from build123d import *

# Parameters (mm, degrees)
SKETCH1_W           = 60
SKETCH1_H           = 25
BOSS_EXTRUDE1_DEPTH = 4
SKETCH3_R           = 1.6
CUT_EXTRUDE1_DEPTH  = 66.122960621
SKETCH4_W           = 60
SKETCH4_H           = 25
SKETCH4_W_2         = 24
SKETCH4_H_2         = 19
SKETCH4_W_3         = 27
BOSS_EXTRUDE2_DEPTH = 30
SKETCH5_R           = 5.25
CUT_EXTRUDE2_DEPTH  = 74.35529974
CUT_EXTRUDE3_REACH  = 75.355
SKETCH6_R           = 1.6
FILLET3_R           = 3
FILLET4_R           = 1
FILLET5_R           = 6
CUT_EXTRUDE4_DEPTH  = 74.35529974
CUT_EXTRUDE5_REACH  = 75.355
CUT_EXTRUDE6_REACH  = 75.355


with BuildPart() as part:
    # Sketch1 → Boss-Extrude1 (new body)
    with BuildSketch(Plane(origin=(0, 0, 0), x_dir=(1, 0, 0), z_dir=(0, 1, 0))):
        with Locations((30, 12.5)):
            Rectangle(SKETCH1_W, SKETCH1_H)
    extrude(amount=BOSS_EXTRUDE1_DEPTH)

    # Sketch3 → Cut-Extrude1 (cut, through all)
    with BuildSketch(Plane(origin=(0, 4, 0), x_dir=(1, 0, 0), z_dir=(0, 1, 0))):
        with Locations(Location((7.5, 17.5, 0), (0, 0, 270))):
            Circle(SKETCH3_R)
        with Locations(Location((22.5, 17.5, 0), (0, 0, 270))):
            Circle(SKETCH3_R)
        with Locations(Location((22.5, 7.5, 0), (0, 0, 270))):
            Circle(SKETCH3_R)
        with Locations(Location((7.5, 7.5, 0), (0, 0, 270))):
            Circle(SKETCH3_R)
    extrude(amount=-CUT_EXTRUDE1_DEPTH, mode=Mode.SUBTRACT)

    # Sketch4 → Boss-Extrude2 (add)
    with BuildSketch(Plane(origin=(0, 4, 0), x_dir=(1, 0, 0), z_dir=(0, 1, 0))):
        with Locations((30, 12.5)):
            Rectangle(SKETCH4_W, SKETCH4_H)
        with Locations((15, 12.5)):
            Rectangle(SKETCH4_W_2, SKETCH4_H_2, mode=Mode.SUBTRACT)
        with Locations((43.5, 12.5)):
            Rectangle(SKETCH4_W_3, SKETCH4_H_2, mode=Mode.SUBTRACT)
    extrude(amount=BOSS_EXTRUDE2_DEPTH)

    # Sketch5 → Cut-Extrude2 (cut, through all)
    with BuildSketch(Plane(origin=(0, 0, -25), x_dir=(-1, 0, 0), z_dir=(0, 0, -1))):
        with Locations((-43.5, 20)):
            Circle(SKETCH5_R)
    extrude(amount=-CUT_EXTRUDE2_DEPTH, mode=Mode.SUBTRACT)

    # Sketch6 → Cut-Extrude3 (cut, up to next)
    with BuildSketch(Plane(origin=(0, 0, -25), x_dir=(-1, 0, 0), z_dir=(0, 0, -1)), mode=Mode.PRIVATE) as cut_extrude3_sk1:
        with Locations((-37.843145751, 14.343145751)):
            Circle(SKETCH6_R)
    cut_extrude3_tool1 = extrude(cut_extrude3_sk1.sketch, amount=-CUT_EXTRUDE3_REACH, mode=Mode.PRIVATE) & part.part
    # Sketch6 → Cut-Extrude3 (cut, up to next)
    with BuildSketch(Plane(origin=(0, 0, -25), x_dir=(-1, 0, 0), z_dir=(0, 0, -1)), mode=Mode.PRIVATE) as cut_extrude3_sk2:
        with Locations((-49.156854249, 14.343145751)):
            Circle(SKETCH6_R)
    cut_extrude3_tool2 = extrude(cut_extrude3_sk2.sketch, amount=-CUT_EXTRUDE3_REACH, mode=Mode.PRIVATE) & part.part
    # Sketch6 → Cut-Extrude3 (cut, up to next)
    with BuildSketch(Plane(origin=(0, 0, -25), x_dir=(-1, 0, 0), z_dir=(0, 0, -1)), mode=Mode.PRIVATE) as cut_extrude3_sk3:
        with Locations((-49.156854249, 25.656854249)):
            Circle(SKETCH6_R)
    cut_extrude3_tool3 = extrude(cut_extrude3_sk3.sketch, amount=-CUT_EXTRUDE3_REACH, mode=Mode.PRIVATE) & part.part
    # Sketch6 → Cut-Extrude3 (cut, up to next)
    with BuildSketch(Plane(origin=(0, 0, -25), x_dir=(-1, 0, 0), z_dir=(0, 0, -1)), mode=Mode.PRIVATE) as cut_extrude3_sk4:
        with Locations((-37.843145751, 25.656854249)):
            Circle(SKETCH6_R)
    cut_extrude3_tool4 = extrude(cut_extrude3_sk4.sketch, amount=-CUT_EXTRUDE3_REACH, mode=Mode.PRIVATE) & part.part
    add(cut_extrude3_tool1.solids().sort_by_distance((37.843146, 14.343146, -25))[0], mode=Mode.SUBTRACT)
    add(cut_extrude3_tool2.solids().sort_by_distance((49.156854, 14.343146, -25))[0], mode=Mode.SUBTRACT)
    add(cut_extrude3_tool3.solids().sort_by_distance((49.156854, 25.656854, -25))[0], mode=Mode.SUBTRACT)
    add(cut_extrude3_tool4.solids().sort_by_distance((37.843146, 25.656854, -25))[0], mode=Mode.SUBTRACT)

    # Fillet3
    fillet3_edges = [part.edges().sort_by_distance(p)[0] for p in [
        (3, 19, -3),
        (27, 19, -3),
        (27, 19, -22),
        (3, 19, -22),
        (57, 19, -3),
        (57, 19, -22),
        (30, 19, -22),
        (30, 19, -3),
    ]]
    fillet(fillet3_edges, radius=FILLET3_R)

    # Fillet4
    fillet4_edges = [part.edges().sort_by_distance(p)[0] for p in [
        (15, 4, -3),
        (15, 4, -22),
        (3, 4, -12.5),
        (27, 4, -12.5),
        (26.121320344, 4, -21.121320344),
        (3.878679656, 4, -21.121320344),
        (3.878679656, 4, -3.878679656),
        (26.121320344, 4, -3.878679656),
        (30, 4, -12.5),
        (43.5, 4, -3),
        (57, 4, -12.5),
        (43.5, 4, -22),
        (30.878679656, 4, -21.121320344),
        (56.121320344, 4, -21.121320344),
        (56.121320344, 4, -3.878679656),
        (30.878679656, 4, -3.878679656),
    ]]
    fillet(fillet4_edges, radius=FILLET4_R)

    # Fillet5
    fillet5_edges = [part.edges().sort_by_distance(p)[0] for p in [
        (0, 17, -25),
        (60, 17, -25),
        (60, 17, 0),
        (0, 17, 0),
    ]]
    fillet(fillet5_edges, radius=FILLET5_R)

    # Sketch7 → Cut-Extrude4 (cut, through all)
    with BuildSketch(Plane(origin=(0, 0, -25), x_dir=(-1, 0, 0), z_dir=(0, 0, -1))):
        with BuildLine():
            Line((-13.4, 26), (-13.4, 34))
            Line((-13.4, 34), (-16.6, 34))
            Line((-16.6, 34), (-16.6, 26))
            ThreePointArc((-16.6, 26), (-15, 24.4), (-13.4, 26))
        make_face()
    extrude(amount=-CUT_EXTRUDE4_DEPTH, mode=Mode.SUBTRACT)

    # Cut-Extrude5: up to this face of the body (flat: up to its plane)
    cut_extrude5_end = Plane(part.part.faces().sort_by_distance((30, 19.5, -12.5))[0])
    # Sketch8 → Cut-Extrude5 (cut, up to the picked face)
    with BuildSketch(Plane.ZY, mode=Mode.PRIVATE) as cut_extrude5_sk1:
        with BuildLine():
            Line((-14.1, 26), (-14.1, 34))
            Line((-14.1, 34), (-10.9, 34))
            Line((-10.9, 34), (-10.9, 26))
            ThreePointArc((-10.9, 26), (-12.5, 24.4), (-14.1, 26))
        make_face()
    cut_extrude5_tool1 = split(extrude(cut_extrude5_sk1.sketch, amount=-CUT_EXTRUDE5_REACH, mode=Mode.PRIVATE), bisect_by=cut_extrude5_end, keep=Keep.BOTH, mode=Mode.PRIVATE)
    add(cut_extrude5_tool1.solids().sort_by(Axis((0, 29.364793, -12.5), (1, 0, 0)))[0], mode=Mode.SUBTRACT)

    # Sketch9 → Cut-Extrude6 (cut, up to next)
    with BuildSketch(Plane(origin=(60, 0, 0), x_dir=(0, 0, -1), z_dir=(1, 0, 0)), mode=Mode.PRIVATE) as cut_extrude6_sk1:
        with BuildLine():
            Line((15, 29), (15, 34))
            Line((15, 34), (10, 34))
            Line((10, 34), (10, 29))
            ThreePointArc((10, 29), (12.5, 26.5), (15, 29))
        make_face()
    cut_extrude6_tool1 = extrude(cut_extrude6_sk1.sketch, amount=-CUT_EXTRUDE6_REACH, mode=Mode.PRIVATE) & part.part
    add(cut_extrude6_tool1.solids().sort_by_distance((60, 30.495896, -12.5))[0], mode=Mode.SUBTRACT)


solid = part.part
Design review of the part built by this model. Coordinates are the model's own, in mm. A direction names the side the tool comes from. Round coordinates to 2 decimals unless told otherwise and drop trailing zeros. Loops run counter-clockwise (first coordinate to the right, second up) from the corner with the lowest first, then second, coordinate; pieces in that order, holes last. Notation, with made-up numbers: M 68.25,11 L 94.25,11 A22 cw 94.25,21 Z; hole C -39,33 d8. An arc over 180 degrees is marked long. Answer as a JSON object with one key per item and string values.
Item 1: We need section A-A on y = 20. State how many separate pieces and enclosed holes the cut face has, and give its area (3 significant figures).
Answer sheet:
{"separate pieces": "2", "enclosed holes": "1", "area": "453 mm^2"}
Item 2: We need section D-D on y = 12. Give the boundary of the cut face in (x, z).
Answer sheet:
{"outline": "M 0,-19 A6 ccw 6,-25 L 54,-25 A6 ccw 60,-19 L 60,-6 A6 ccw 54,0 L 6,0 A6 ccw 0,-6 Z; hole M 3,-19 A3 ccw 6,-22 L 24,-22 A3 ccw 27,-19 L 27,-6 A3 ccw 24,-3 L 6,-3 A3 ccw 3,-6 Z; hole M 30,-19 A3 ccw 33,-22 L 54,-22 A3 ccw 57,-19 L 57,-6 A3 ccw 54,-3 L 33,-3 A3 ccw 30,-6 Z"}
Item 3: Clearance check with flat-ended pins moving along their axes: P1, Ø4, axis at x = 37.84, y = 14.34, coming from the -Z side; P2, Ø3.5, axis at y = 31.5, z = -1, coming from the +X side; P3, Ø3.5, axis at x = 1.5, y = 29.5, coming from the -Z side; P4, Ø2.5, axis at y = 29, z = -1, coming from the -X side. State where each tip first meets the part, or that it passes through.
Answer sheet:
{"P1": "stops at z = -25", "P2": "stops at x = 59.04", "P3": "stops at z = -24.33", "P4": "stops at x = 1.32"}
Item 4: Wall thickness on L1, parallel to X at y = 15, z = -13; L2, parallel to X at y = 3, z = -7.5; L3, parallel to Z at x = 22, y = 28: over which ranges is each line inside the solid? List them lowest first. Write a range as from..to.
Answer sheet:
{"L1": "x = 0..3, 27..30, 57..60", "L2": "x = 0..5.9, 9.1..20.9, 24.1..60", "L3": "z = -25..-22, -3..0"}
Item 5: We need section C-C on z = -17.5. Give the boundary of the cut face in (x, y), and give its area (3 significant figures).
Answer sheet:
{"outline": "M 0,0 L 5.9,0 L 5.9,4 L 4,4 A1 cw 3,5 L 3,34 L 0,34 Z; M 9.1,0 L 20.9,0 L 20.9,4 L 9.1,4 Z; M 24.1,0 L 60,0 L 60,34 L 57,34 L 57,5 A1 cw 56,4 L 31,4 A1 cw 30,5 L 30,34 L 27,34 L 27,5 A1 cw 26,4 L 24.1,4 Z", "area": "485 mm^2"}
Item 6: We need section B-B on x = 7.5. Give the boundary of the cut face in (y, z).
Answer sheet:
{"outline": "M 0,-25 L 34,-25 L 34,-22 L 5,-22 A1 cw 4,-21 L 4,-19.1 L 0,-19.1 Z; M 0,-15.9 L 4,-15.9 L 4,-9.1 L 0,-9.1 Z; M 0,-5.9 L 4,-5.9 L 4,-4 A1 cw 5,-3 L 34,-3 L 34,0 L 0,0 Z"}
Item 7: Machinability: for faces 1 (the flat face through (38, 34, -23)), 2 (the flat face through (30, 17, -25)), 3 (the cylindrical face through (47.63, 14.82, -23.52)), 4 (the flat face through (15, 4, -13)), 5 (the flat face through (59, 32, -10)), which of the approach directions +Z, -Z, +X, -X, +Y, -Y give a long, thin tool a straight path to every point of the face, cutting with its end or side? Answer none if there is none.
Answer sheet:
{"face 1": "+Z, -Z, +X, -X, +Y", "face 2": "-Z, +X, -X, +Y, -Y", "face 3": "-Z", "face 4": "+Y", "face 5": "+X, +Y"}
Item 8: The part is to be moulded in two halves that separate along X. For faces 6 (the cylindrical face through (15, 24.4, -23.5)), 7 (the flat face through (39, 16, -3)), 8 (the flat face through (5, 34, -22)), say which applies: pulls with the +X half, pulls with the -X half, needs draft (parallel to the pull), parting line crosses it, or undercut.
Answer sheet:
{"face 6": "undercut", "face 7": "undercut", "face 8": "needs draft"}
